from build123d import *

# Parameters (mm, degrees)
CUT_EXTRUDE1_START = -12.7
SKETCH3_R          = 3.556
CUT_EXTRUDE1_DEPTH = 29.918152
SKETCH4_R          = 2.0828
CUT_EXTRUDE2_DEPTH = 12.7
CIRPATTERN1_COUNT  = 8


with BuildPart() as part:
    # Sketch2 → Revolve1 (revolve)
    with BuildSketch(Plane.XY, mode=Mode.PRIVATE) as revolve1_sk:
        with BuildLine():
            Line((61.871733, 7.1480426), (51.29041327, 5.055001066))
            ThreePointArc((51.29041327, 5.055001066), (51.046380141, 5.018882817), (50.8, 5.0064924))
            ThreePointArc((50.8, 5.0064924), (49.841678346, 5.196168991), (49.0299248, 5.7396888))
            Line((49.0299248, 5.7396888), (38.3808732, 16.3887404))
            ThreePointArc((38.3808732, 16.3887404), (35.432006503, 18.359111266), (31.953581, 19.051016))
            Line((31.953581, 19.051016), (25.603581, 19.051016))
            Line((25.603581, 19.051016), (25.603581, 22.225))
            Line((25.603581, 22.225), (19.253581, 22.225))
            Line((19.253581, 22.225), (19.253581, 31.115))
            Line((19.253581, 31.115), (20.351883229, 31.115))
            ThreePointArc((20.351883229, 31.115), (34.230433921, 28.832379737), (46.646836686, 22.225))
            ThreePointArc((46.646836686, 22.225), (48.658911913, 21.154275625), (50.907927879, 20.784377533))
            Line((50.907927879, 20.784377533), (61.871733, 20.784377533))
            Line((61.871733, 20.784377533), (61.871733, 7.1480426))
        make_face()
    revolve(revolve1_sk.sketch.rotate(Axis((0, 0, 0), (1, 0, 0)), 90), axis=Axis((0, 0, 0), (1, 0, 0)))

    # Sketch3 → Cut-Extrude1 (cut)
    with BuildSketch(Plane.ZY.offset(-19.253581).offset(CUT_EXTRUDE1_START)):
        with Locations((0, 26.67)):
            Circle(SKETCH3_R)
    cut_extrude1 = extrude(amount=-CUT_EXTRUDE1_DEPTH, mode=Mode.SUBTRACT)

    # Sketch4 → Cut-Extrude2 (cut)
    with BuildSketch(Plane(origin=(31.953581, 0, 0), x_dir=(0, 0, -1), z_dir=(1, 0, 0))):
        with Locations((0, 26.67)):
            Circle(SKETCH4_R)
    cut_extrude2 = extrude(amount=-CUT_EXTRUDE2_DEPTH, mode=Mode.SUBTRACT)

    # CirPattern1: Cut-Extrude1, Cut-Extrude2 ×8 about axis
    cirpattern1_axis = Axis((0, 0, 0), (1, 0, 0))
    add([cut_extrude1.rotate(cirpattern1_axis, i * 360 / CIRPATTERN1_COUNT) for i in range(1, CIRPATTERN1_COUNT)], mode=Mode.SUBTRACT)
    add([cut_extrude2.rotate(cirpattern1_axis, i * 360 / CIRPATTERN1_COUNT) for i in range(1, CIRPATTERN1_COUNT)], mode=Mode.SUBTRACT)


solid = part.part
Could you check a few things on this model? Use its own coordinates, in mm. A direction names the side the tool comes from. Give positions to 0.01 mm unless a question says otherwise; leave off trailing zeros. Return JSON: item names as keys, results as strings.
1. On a 3-axis mill with a long thin cutter (end or side, diameter ignored), from which of +Z, -Z, +X, -X, +Y, -Y can I reach the whole of each face in a straight line? I mean faces 1 (the cylindrical face through (25.69, 0.96, 24.82)), 2 (the cylindrical face through (37.11, -16.26, 16.43)). Say none if no direction works.
Answer list:
{"face 1": "+X, -X", "face 2": "+X"}
2. Imagine slicing it at A-A on y = 0. Give the number of separate pieces and of enclosed holes in the cut face, then the cut area to 3 significant figures.
Answer list:
{"separate pieces": "4", "enclosed holes": "0", "area": "841 mm2"}
3. I need wall thicknesses on line 1 (Y direction, x = 28.75, z = 0); line 2 (Y direction, x = 25, z = 19.5); line 3 (Z direction, x = 22, y = 11). Which ranges of each line are inside material? Lowest first, please. Write a range as from..to.
Answer list:
{"line 1": "y = -30.29..-28.75, -24.59..-19.05, 19.05..24.59, 28.75..30.29", "line 2": "y = -23.92..-20.84, -16.88..-10.66, 10.66..16.88, 20.84..23.92", "line 3": "z = -29.07..-19.31, 19.31..29.07"}
4. For pin 1 Ø5 at (x, z) = (28, -14.5) entering from -Y; pin 2 Ø4 at (y, z) = (10.5, 0.5) entering from -X; pin 3 Ø6 at (y, z) = (-10, -16) entering from -X; pin 4 Ø2 at (y, z) = (19.5, -19.5) entering from +X, each with a flat end and sliding along its axis, tell me the tip position at first contact or that it passes through.
Answer list:
{"pin 1": "stops at y = -28.06", "pin 2": "stops at x = 42.26", "pin 3": "stops at x = 25.6", "pin 4": "passes through"}
